Design review of the part built by this model. Coordinates are the model's own, in mm. Face numbers are marked on the shaded views. Give positions to 0.01 mm unless a question says otherwise; leave off trailing zeros. Write each loop counter-clockwise with the first axis right and the second up, starting at its lowest first coordinate (ties: lowest second). Pieces come first, ordered by that corner, then holes. Notation, with made-up numbers: (68.5, 50) -> (121.5, 50) arc R14 cw to (121.5, 63) -> close; hole circle Ø7 at (56, -10.75). An arc over 180 degrees is marked (long way). Use CSV: the item, a comma, the result in double quotes.
```python
from build123d import *

# Parameters (mm, degrees)
SKETCH_1_W                 = 200.502
SKETCH_1_H                 = 67.152
EXTRUDE_2_DEPTH            = 34.5
SHELL_3_T                  = -3
SHELL_3_THICKNESS_2_FACE_W = 194.502
SHELL_3_THICKNESS_2_FACE_H = 31.5
SHELL_3_THICKNESS_2_DEPTH  = 7
SHELL_3_THICKNESS_3_FACE_W = 31.5
SHELL_3_THICKNESS_3_FACE_H = 54.152
SHELL_3_THICKNESS_3_DEPTH  = 7
SHELL_3_THICKNESS_4_FACE_W = 31.5
SHELL_3_THICKNESS_4_FACE_H = 54.152
SHELL_3_THICKNESS_4_DEPTH  = 7
SHELL_3_THICKNESS_5_FACE_W = 180.502
SHELL_3_THICKNESS_5_FACE_H = 31.5
SHELL_3_THICKNESS_5_DEPTH  = 7


with BuildPart() as part:
    # 草图1 → 凸台-拉伸2 (new body)
    with BuildSketch(Plane.XY):
        Rectangle(SKETCH_1_W, SKETCH_1_H)
    extrude(amount=EXTRUDE_2_DEPTH)

    # 抽壳3
    shell_3_openings = [part.faces().sort_by_distance(p)[0] for p in [
        (0, 0, 34.5),
    ]]
    offset(amount=SHELL_3_T, openings=shell_3_openings, kind=Kind.INTERSECTION)

    # 抽壳3 thickness 2 face (on inner face of the shell) → 抽壳3 thickness 2 (add)
    with BuildSketch(Plane(origin=(0, 30.576, 18.75), x_dir=(1, 0, 0), z_dir=(0, 1, 0))):
        Rectangle(SHELL_3_THICKNESS_2_FACE_W, SHELL_3_THICKNESS_2_FACE_H)
    extrude(amount=-SHELL_3_THICKNESS_2_DEPTH)

    # 抽壳3 thickness 3 face (on inner face of the shell) → 抽壳3 thickness 3 (add)
    with BuildSketch(Plane(origin=(97.251, -3.5, 18.75), x_dir=(0, 0, 1), z_dir=(1, 0, 0))):
        Rectangle(SHELL_3_THICKNESS_3_FACE_W, SHELL_3_THICKNESS_3_FACE_H)
    extrude(amount=-SHELL_3_THICKNESS_3_DEPTH)

    # 抽壳3 thickness 4 face (on inner face of the shell) → 抽壳3 thickness 4 (add)
    with BuildSketch(Plane(origin=(-97.251, -3.5, 18.75), x_dir=(0, 0, -1), z_dir=(-1, 0, 0))):
        Rectangle(SHELL_3_THICKNESS_4_FACE_W, SHELL_3_THICKNESS_4_FACE_H)
    extrude(amount=-SHELL_3_THICKNESS_4_DEPTH)

    # 抽壳3 thickness 5 face (on inner face of the shell) → 抽壳3 thickness 5 (add)
    with BuildSketch(Plane(origin=(0, -30.576, 18.75), x_dir=(-1, 0, 0), z_dir=(0, -1, 0))):
        Rectangle(SHELL_3_THICKNESS_5_FACE_W, SHELL_3_THICKNESS_5_FACE_H)
    extrude(amount=-SHELL_3_THICKNESS_5_DEPTH)


solid = part.part
```
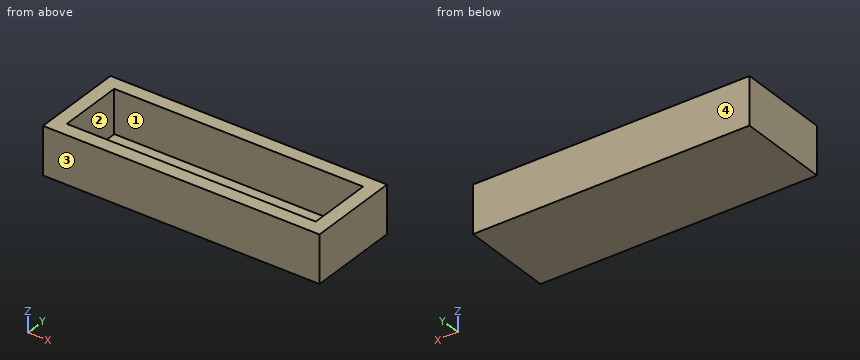
(1) Take a section at B-B (y = 11). Write out the cut boundary in (x, z), then the cut area to 3 significant figures.
Established:
outline,"(-100.25, 0) -> (100.25, 0) -> (100.25, 34.5) -> (90.25, 34.5) -> (90.25, 3) -> (-90.25, 3) -> (-90.25, 34.5) -> (-100.25, 34.5) -> close"
area,"1,230 mm2"
(2) Take a section at A-A (z = 24.5). Write out the cut boundary in (x, y), then the cut area to 3 significant figures.
Established:
outline,"(-100.25, -33.58) -> (100.25, -33.58) -> (100.25, 33.58) -> (-100.25, 33.58) -> close; hole (-90.25, -23.58) -> (90.25, -23.58) -> (90.25, 23.58) -> (-90.25, 23.58) -> close"
area,"4,950 mm2"
(3) For line 1 along Y through (x, z) = (73, 29.5); line 2 along X through (y, z) = (14, 13); line 3 along Z through (x, y) = (62.5, 3), list the stretches that pass through material, from the lowest coordinate up. Write a range as [from, to].
Established:
line 1,"y = [-33.58, -23.58], [23.58, 33.58]"
line 2,"x = [-100.25, -90.25], [90.25, 100.25]"
line 3,"z = [0, 3]"
(4) Clearance check with flat-ended pins moving along their axes: pin 1 (6 mm diameter, centred on x = 60.5, y = 23, fed in from -Z); pin 2 (14 mm diameter, centred on x = -9, y = 10, fed in from +Z). State where each tip first meets the part, or that it passes through.
Established:
pin 1,"stops at z = 0"
pin 2,"stops at z = 3"
(5) Take a section at C-C (x = 11). Write out the cut boundary in (y, z), then the cut area to 3 significant figures.
Established:
outline,"(-33.58, 0) -> (33.58, 0) -> (33.58, 34.5) -> (23.58, 34.5) -> (23.58, 3) -> (-23.58, 3) -> (-23.58, 34.5) -> (-33.58, 34.5) -> close"
area,"831 mm2"
(6) Mouldability with a two-part tool opening along Y and no side actions: class the marked faces 1, 2, 3 and 4 as +Y half, -Y half, draft (parallel to the pull), parting line (faces both ways), or undercut.
Established:
face 1,"undercut"
face 2,"undercut"
face 3,"-Y half"
face 4,"+Y half"
